Model file for the job. Use its own axes, mm. A direction names the side the tool comes from. Coordinates: 2 decimals unless noted, no trailing zeros. Write each loop counter-clockwise with the first axis right and the second up, starting at its lowest first coordinate (ties: lowest second). Pieces come first, ordered by that corner, then holes. Notation, with made-up numbers: M 79.25,88 L 125.25,88 A10 ccw 125.25,103 Z; hole C 9,31.25 d4. An arc over 180 degrees is marked long. Use CSV: the item, a comma, the result in double quotes. Start each with the question number.
from build123d import *

# Parameters (mm, degrees)
SKETCH1_W                   = 33
SKETCH1_H                   = 33
BOSS_EXTRUDE1_DEPTH         = 65
FILLET1_R                   = 1
CUT_EXTRUDE2_START          = -30
CUT_EXTRUDE2_OUTLINE_R      = 8
CUT_EXTRUDE2_DEPTH          = 30
TAP_DRILL_FOR_M3_TAP1_D     = 2.5
TAP_DRILL_FOR_M3_TAP1_DEPTH = 20
TAP_DRILL_FOR_M3_TAP1_TIP   = 0.751075774
CUT_EXTRUDE5_REACH          = 82.019
SKETCH6_W                   = 2
SKETCH6_H                   = 1.3
CIRPATTERN1_COUNT           = 3
CIRPATTERN1_ANGLE           = 180
CIRPATTERN1_COPY_1_REACH    = 82.019
CIRPATTERN1_COPY_1_SKETCH_W = 2
CIRPATTERN1_COPY_1_SKETCH_H = 1.3
CIRPATTERN1_COPY_2_REACH    = 82.019
CIRPATTERN1_COPY_2_SKETCH_W = 2
CIRPATTERN1_COPY_2_SKETCH_H = 1.3


# Read off the part's stored shape, not the designer's step: Cut-Extrude2
with BuildPart() as part:
    # Sketch1 → Boss-Extrude1 (new body)
    with BuildSketch(Plane.XY):
        with Locations((16.5, 16.5)):
            Rectangle(SKETCH1_W, SKETCH1_H)
    extrude(amount=BOSS_EXTRUDE1_DEPTH)

    # Fillet1
    fillet1_edges = [part.edges().sort_by_distance(p)[0] for p in [
        (0, 33, 32.5),
        (33, 33, 32.5),
        (33, 0, 32.5),
        (0, 0, 32.5),
    ]]
    fillet(fillet1_edges, radius=FILLET1_R)

    # Cut-Extrude2 outline → Cut-Extrude2 (cut)
    with BuildSketch(Plane.XY.offset(65).offset(CUT_EXTRUDE2_START)):
        with Locations((16.5, 16.5)):
            Circle(CUT_EXTRUDE2_OUTLINE_R)
    extrude(amount=CUT_EXTRUDE2_DEPTH, mode=Mode.SUBTRACT)

    # Tap Drill for M3 Tap1
    with Locations(Plane(origin=(0, 0, 0), x_dir=(0, -1, 0), z_dir=(-1, 0, 0))):
        with Locations((-16.5, 55.5), (-16.5, 48), (-16.5, 30.5), (-16.5, 18)):
            Hole(TAP_DRILL_FOR_M3_TAP1_D / 2, depth=TAP_DRILL_FOR_M3_TAP1_DEPTH)
            with Locations((0, 0, -(TAP_DRILL_FOR_M3_TAP1_DEPTH + TAP_DRILL_FOR_M3_TAP1_TIP / 2))):  # 118° drill point
                Cone(0, TAP_DRILL_FOR_M3_TAP1_D / 2, TAP_DRILL_FOR_M3_TAP1_TIP, mode=Mode.SUBTRACT)

    # Sketch6 → Cut-Extrude5 (cut, up to next)
    with BuildSketch(Plane.XY.offset(65), mode=Mode.PRIVATE) as cut_extrude5_sk1:
        with Locations((5, 32.35)):
            Rectangle(SKETCH6_W, SKETCH6_H)
    cut_extrude5_tool1 = extrude(cut_extrude5_sk1.sketch, amount=-CUT_EXTRUDE5_REACH, mode=Mode.PRIVATE) & part.part
    # Sketch6 → Cut-Extrude5 (cut, up to next)
    with BuildSketch(Plane.XY.offset(65), mode=Mode.PRIVATE) as cut_extrude5_sk2:
        with Locations((7.5, 32.35)):
            Rectangle(SKETCH6_W, SKETCH6_H)
    cut_extrude5_tool2 = extrude(cut_extrude5_sk2.sketch, amount=-CUT_EXTRUDE5_REACH, mode=Mode.PRIVATE) & part.part
    # Sketch6 → Cut-Extrude5 (cut, up to next)
    with BuildSketch(Plane.XY.offset(65), mode=Mode.PRIVATE) as cut_extrude5_sk3:
        with Locations((10, 32.35)):
            Rectangle(SKETCH6_W, SKETCH6_H)
    cut_extrude5_tool3 = extrude(cut_extrude5_sk3.sketch, amount=-CUT_EXTRUDE5_REACH, mode=Mode.PRIVATE) & part.part
    # Sketch6 → Cut-Extrude5 (cut, up to next)
    with BuildSketch(Plane.XY.offset(65), mode=Mode.PRIVATE) as cut_extrude5_sk4:
        with Locations((12.5, 32.35)):
            Rectangle(SKETCH6_W, SKETCH6_H)
    cut_extrude5_tool4 = extrude(cut_extrude5_sk4.sketch, amount=-CUT_EXTRUDE5_REACH, mode=Mode.PRIVATE) & part.part
    cut_extrude5_1 = cut_extrude5_tool1.solids().sort_by_distance((5, 32.35, 65))[0]
    add(cut_extrude5_1, mode=Mode.SUBTRACT)
    cut_extrude5_2 = cut_extrude5_tool2.solids().sort_by_distance((7.5, 32.35, 65))[0]
    add(cut_extrude5_2, mode=Mode.SUBTRACT)
    cut_extrude5_3 = cut_extrude5_tool3.solids().sort_by_distance((10, 32.35, 65))[0]
    add(cut_extrude5_3, mode=Mode.SUBTRACT)
    cut_extrude5_4 = cut_extrude5_tool4.solids().sort_by_distance((12.5, 32.35, 65))[0]
    add(cut_extrude5_4, mode=Mode.SUBTRACT)
    cut_extrude5 = cut_extrude5_1 + cut_extrude5_2 + cut_extrude5_3 + cut_extrude5_4  # Cut-Extrude5 as one shape, for the pattern or mirror that repeats it

    # Mirror2: Cut-Extrude5 across plane
    add(cut_extrude5.mirror(Plane(origin=(16.5, 0, 0), x_dir=(0, 0, 1), z_dir=(1, 0, 0))), mode=Mode.SUBTRACT)

    # CirPattern1: Cut-Extrude5 ×3 about axis
    cirpattern1_axis = Axis((16.5, 16.5, 0), (0, 0, -1))
    for i in range(1, CIRPATTERN1_COUNT):
        add(cut_extrude5.rotate(cirpattern1_axis, i * CIRPATTERN1_ANGLE / (CIRPATTERN1_COUNT - 1)), mode=Mode.SUBTRACT)

    # CirPattern1 copy 1 sketch → CirPattern1 copy 1 (cut, up to next)
    with BuildSketch(Plane(origin=(0, 0, 65), x_dir=(0, 1, 0), z_dir=(0, 0, 1)), mode=Mode.PRIVATE) as cirpattern1_copy_1_sk1:
        with Locations((5, -32.35)):
            Rectangle(CIRPATTERN1_COPY_1_SKETCH_W, CIRPATTERN1_COPY_1_SKETCH_H)
    cirpattern1_copy_1_tool1 = extrude(cirpattern1_copy_1_sk1.sketch, amount=-CIRPATTERN1_COPY_1_REACH, mode=Mode.PRIVATE) & part.part
    # CirPattern1 copy 1 sketch → CirPattern1 copy 1 (cut, up to next)
    with BuildSketch(Plane(origin=(0, 0, 65), x_dir=(0, 1, 0), z_dir=(0, 0, 1)), mode=Mode.PRIVATE) as cirpattern1_copy_1_sk2:
        with Locations((7.5, -32.35)):
            Rectangle(CIRPATTERN1_COPY_1_SKETCH_W, CIRPATTERN1_COPY_1_SKETCH_H)
    cirpattern1_copy_1_tool2 = extrude(cirpattern1_copy_1_sk2.sketch, amount=-CIRPATTERN1_COPY_1_REACH, mode=Mode.PRIVATE) & part.part
    # CirPattern1 copy 1 sketch → CirPattern1 copy 1 (cut, up to next)
    with BuildSketch(Plane(origin=(0, 0, 65), x_dir=(0, 1, 0), z_dir=(0, 0, 1)), mode=Mode.PRIVATE) as cirpattern1_copy_1_sk3:
        with Locations((10, -32.35)):
            Rectangle(CIRPATTERN1_COPY_1_SKETCH_W, CIRPATTERN1_COPY_1_SKETCH_H)
    cirpattern1_copy_1_tool3 = extrude(cirpattern1_copy_1_sk3.sketch, amount=-CIRPATTERN1_COPY_1_REACH, mode=Mode.PRIVATE) & part.part
    # CirPattern1 copy 1 sketch → CirPattern1 copy 1 (cut, up to next)
    with BuildSketch(Plane(origin=(0, 0, 65), x_dir=(0, 1, 0), z_dir=(0, 0, 1)), mode=Mode.PRIVATE) as cirpattern1_copy_1_sk4:
        with Locations((12.5, -32.35)):
            Rectangle(CIRPATTERN1_COPY_1_SKETCH_W, CIRPATTERN1_COPY_1_SKETCH_H)
    cirpattern1_copy_1_tool4 = extrude(cirpattern1_copy_1_sk4.sketch, amount=-CIRPATTERN1_COPY_1_REACH, mode=Mode.PRIVATE) & part.part
    add(cirpattern1_copy_1_tool1.solids().sort_by_distance((32.35, 5, 65))[0], mode=Mode.SUBTRACT)
    add(cirpattern1_copy_1_tool2.solids().sort_by_distance((32.35, 7.5, 65))[0], mode=Mode.SUBTRACT)
    add(cirpattern1_copy_1_tool3.solids().sort_by_distance((32.35, 10, 65))[0], mode=Mode.SUBTRACT)
    add(cirpattern1_copy_1_tool4.solids().sort_by_distance((32.35, 12.5, 65))[0], mode=Mode.SUBTRACT)

    # CirPattern1 copy 2 sketch → CirPattern1 copy 2 (cut, up to next)
    with BuildSketch(Plane(origin=(0, 33, 65), x_dir=(1, 0, 0), z_dir=(0, 0, 1)), mode=Mode.PRIVATE) as cirpattern1_copy_2_sk1:
        with Locations((5, -32.35)):
            Rectangle(CIRPATTERN1_COPY_2_SKETCH_W, CIRPATTERN1_COPY_2_SKETCH_H)
    cirpattern1_copy_2_tool1 = extrude(cirpattern1_copy_2_sk1.sketch, amount=-CIRPATTERN1_COPY_2_REACH, mode=Mode.PRIVATE) & part.part
    # CirPattern1 copy 2 sketch → CirPattern1 copy 2 (cut, up to next)
    with BuildSketch(Plane(origin=(0, 33, 65), x_dir=(1, 0, 0), z_dir=(0, 0, 1)), mode=Mode.PRIVATE) as cirpattern1_copy_2_sk2:
        with Locations((7.5, -32.35)):
            Rectangle(CIRPATTERN1_COPY_2_SKETCH_W, CIRPATTERN1_COPY_2_SKETCH_H)
    cirpattern1_copy_2_tool2 = extrude(cirpattern1_copy_2_sk2.sketch, amount=-CIRPATTERN1_COPY_2_REACH, mode=Mode.PRIVATE) & part.part
    # CirPattern1 copy 2 sketch → CirPattern1 copy 2 (cut, up to next)
    with BuildSketch(Plane(origin=(0, 33, 65), x_dir=(1, 0, 0), z_dir=(0, 0, 1)), mode=Mode.PRIVATE) as cirpattern1_copy_2_sk3:
        with Locations((10, -32.35)):
            Rectangle(CIRPATTERN1_COPY_2_SKETCH_W, CIRPATTERN1_COPY_2_SKETCH_H)
    cirpattern1_copy_2_tool3 = extrude(cirpattern1_copy_2_sk3.sketch, amount=-CIRPATTERN1_COPY_2_REACH, mode=Mode.PRIVATE) & part.part
    # CirPattern1 copy 2 sketch → CirPattern1 copy 2 (cut, up to next)
    with BuildSketch(Plane(origin=(0, 33, 65), x_dir=(1, 0, 0), z_dir=(0, 0, 1)), mode=Mode.PRIVATE) as cirpattern1_copy_2_sk4:
        with Locations((12.5, -32.35)):
            Rectangle(CIRPATTERN1_COPY_2_SKETCH_W, CIRPATTERN1_COPY_2_SKETCH_H)
    cirpattern1_copy_2_tool4 = extrude(cirpattern1_copy_2_sk4.sketch, amount=-CIRPATTERN1_COPY_2_REACH, mode=Mode.PRIVATE) & part.part
    add(cirpattern1_copy_2_tool1.solids().sort_by_distance((5, 0.65, 65))[0], mode=Mode.SUBTRACT)
    add(cirpattern1_copy_2_tool2.solids().sort_by_distance((7.5, 0.65, 65))[0], mode=Mode.SUBTRACT)
    add(cirpattern1_copy_2_tool3.solids().sort_by_distance((10, 0.65, 65))[0], mode=Mode.SUBTRACT)
    add(cirpattern1_copy_2_tool4.solids().sort_by_distance((12.5, 0.65, 65))[0], mode=Mode.SUBTRACT)


solid = part.part
1) Two-plate mould, pull along Z, no slides. Class faces 4 (the face through (20.62, 16.4, 17.81)), 5 (the face through (11.5, 32, 33)), 6 (the face through (16, 17, 0)): pulls with the +Z half, pulls with the -Z half, needs draft (parallel to the pull), parting line crosses it, or undercut.
2) Band-saw the part on A-A on x = 16.5. List the corners of the cut face in (y, z), then the cut area to 3 significant figures.
3) Wall check: L1, parallel to Z at x = 6, y = 16.5; L2, parallel to Z at x = 7, y = 15.5; L3, parallel to Y at x = 5, z = 48. Give the ranges that are in metal, low to high. Write a range as [from, to].
4) Tool access for faces 1 (the face through (32, 11, 33)), 2 (the face through (5, 31.7, 33)), 3 (the face through (10, 1.3, 33)): list every direction of +Z, -Z, +X, -X, +Y, -Y with a clear straight run to the whole face (end or side of a thin tool).
5) Drop flat-ended pins along their axis: P1, Ø0.6, axis at x = 32.5, z = 22.5, coming from the +Y side; P2, Ø0.6, axis at y = 32.5, z = 32.5, coming from the -X side; P3, Ø0.6, axis at y = 0.5, z = 35.5, coming from the +X side. Give the stop position or say it passes through.
Findings below:
1,face 4,"undercut"
1,face 5,"needs draft"
1,face 6,"pulls with the -Z half"
2,outline,"M 0,0 L 33,0 L 33,65 L 24.5,65 L 24.5,35 L 8.5,35 L 8.5,65 L 0,65 Z; hole C 16.5,18 d2.5; hole C 16.5,30.5 d2.5"
2,area,"1,660 mm2"
3,L1,"z = [0, 16.75], [19.25, 29.25], [31.75, 46.75], [49.25, 54.25], [56.75, 65]"
3,L2,"z = [0, 17.25], [18.75, 29.75], [31.25, 47.25], [48.75, 54.75], [56.25, 65]"
3,L3,"y = [1.3, 15.25], [17.75, 31.7]"
4,face 1,"+Z, -Z, +X"
4,face 2,"+Z, -Z, +Y"
4,face 3,"+Z, -Z, -Y"
5,P1,"stops at y = 32.98"
5,P2,"stops at x = 0.02"
5,P3,"stops at x = 32.98"
